```python
from build123d import *

# Parameters (mm, degrees)
SKETCH1_R           = 11.43
BOSS_EXTRUDE1_DEPTH = 1.524
BOSS_EXTRUDE2_DEPTH = 12.954
CHAMFER1_SIZE       = 3.175
CHAMFER2_SIZE       = 0.762
SKETCH3_R           = 1.8415
BOSS_EXTRUDE3_DEPTH = 5.08


with BuildPart() as part:
    # Sketch1 → Boss-Extrude1 (new body)
    with BuildSketch(Plane.XY):
        Circle(SKETCH1_R)
    extrude(amount=-BOSS_EXTRUDE1_DEPTH)

    # Sketch2 → Boss-Extrude2 (add)
    with BuildSketch(Plane(origin=(0, 0, -1.524), x_dir=(-1, 0, 0), z_dir=(0, 0, -1))):
        with BuildLine():
            Line((-2.052467985, 4.297532015), (4.297532015, -2.052467985))
            ThreePointArc((4.297532015, -2.052467985), (-3.367596045, -3.367596045), (-2.052467985, 4.297532015))
        make_face()
    extrude(amount=BOSS_EXTRUDE2_DEPTH)

    # Chamfer1
    chamfer1_edges = [part.edges().sort_by_distance(p)[0] for p in [
        (-1.122532015, 1.122532015, -14.478),
    ]]
    chamfer(chamfer1_edges, length=CHAMFER1_SIZE)

    # Chamfer2
    chamfer2_edges = [part.edges().sort_by_distance(p)[0] for p in [
        (3.367596045, -3.367596045, -14.478),
    ]]
    chamfer(chamfer2_edges, length=CHAMFER2_SIZE)

    # Sketch3 → Boss-Extrude3 (add)
    with BuildSketch(Plane.XY):
        with Locations((6.868507686, 5.763362266)):
            Circle(SKETCH3_R)
    extrude(amount=BOSS_EXTRUDE3_DEPTH)


solid = part.part
```
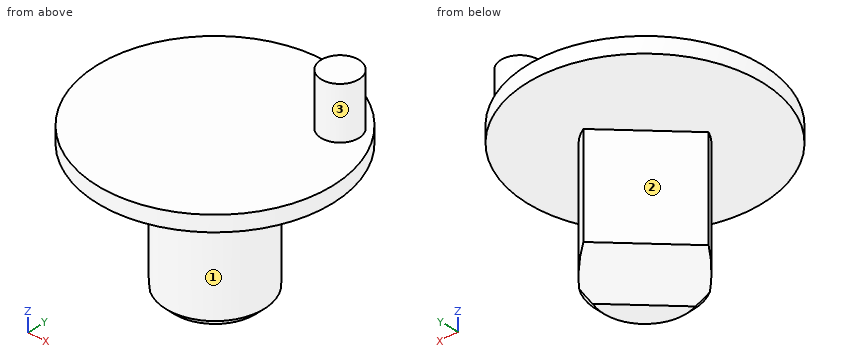
Could you check a few things on this model? Use its own coordinates, in mm. Face numbers are marked on the shaded views. A direction names the side the tool comes from. Give positions to 0.01 mm unless a question says otherwise; leave off trailing zeros. Loops run counter-clockwise (first coordinate to the right, second up) from the corner with the lowest first, then second, coordinate; pieces in that order, holes last. Notation, with made-up numbers: (12, -27.5) - (44, -27.5) arc R14 cw to (44, -16.5) - close; hole circle Ø1 at (-5, 35). An arc over 180 degrees is marked (long way). Answer in a Markdown table with one row per item. Add a question column.
Q1. If we section it at B-B (z = -5): List the corners of the cut face in (x, y) for me (1 decimal).
Q2. Please list where these lines run through material, in increasing order: L1, parallel to Z at x = -0.25, y = -9.5; L2, parallel to Z at x = 6.75, y = 7.5; L3, parallel to Y at x = 0.5, z = -10. Write a range as from..to.
Q3. For pin 1 (4 mm diameter, centred on x = -1, y = 6, fed in from +Z); pin 2 (3 mm diameter, centred on y = -4, z = -4.5, fed in from +X); pin 3 (1 mm diameter, centred on x = -4.5, y = 2.5, fed in from -Z), each with a flat end and sliding along its axis, tell me the tip position at first contact or that it passes through.
Q4. Which directions (+Z, -Z, +X, -X, +Y, -Y) give clear straight access to the entire face, cutting with the end or side of a thin tool? Please do the marked faces 1, 2 and 3.
Q5. If we section it at D-D (x = -3.5): List the corners of the cut face in (y, z) for me.
Q6. If we section it at C-C (y = 0): List the corners of the cut face in (x, z) for me.
Q7. If we section it at A-A (x = 0): List the corners of the cut face in (y, z) for me, plus the area to 3 significant figures.
The answers:
| question | item | result |
|---|---|---|
| 1 | outline | (-4.3, -2.1) arc R4.8 ccw (long way) to (2.1, 4.3) - close |
| 2 | L1 | z = -1.52..0 |
| 2 | L2 | z = -1.52..5.08 |
| 2 | L3 | y = -4.74..2.75 |
| 3 | pin 1 | stops at z = 0 |
| 3 | pin 2 | stops at x = 4.05 |
| 3 | pin 3 | stops at z = -1.52 |
| 4 | face 1 | -Z |
| 4 | face 2 | -Z, -X, +Y |
| 4 | face 3 | +Z |
| 5 | outline | (-10.88, -1.52) - (-3.23, -1.52) - (-3.23, -12.7) - (-1.25, -11.3) - (-1.25, -1.52) - (10.88, -1.52) - (10.88, 0) - (-10.88, 0) - close |
| 6 | outline | (-11.43, -1.52) - (-2.25, -1.52) - (-2.25, -11.3) - (2.25, -14.48) - (4, -14.48) - (4.76, -13.72) - (4.76, -1.52) - (11.43, -1.52) - (11.43, 0) - (-11.43, 0) - close |
| 7 | outline | (-11.43, -1.52) - (-4.76, -1.52) - (-4.76, -13.72) - (-4, -14.48) - (-2.25, -14.48) - (2.25, -11.3) - (2.25, -1.52) - (11.43, -1.52) - (11.43, 0) - (-11.43, 0) - close |
| 7 | area | 118 mm^2 |
